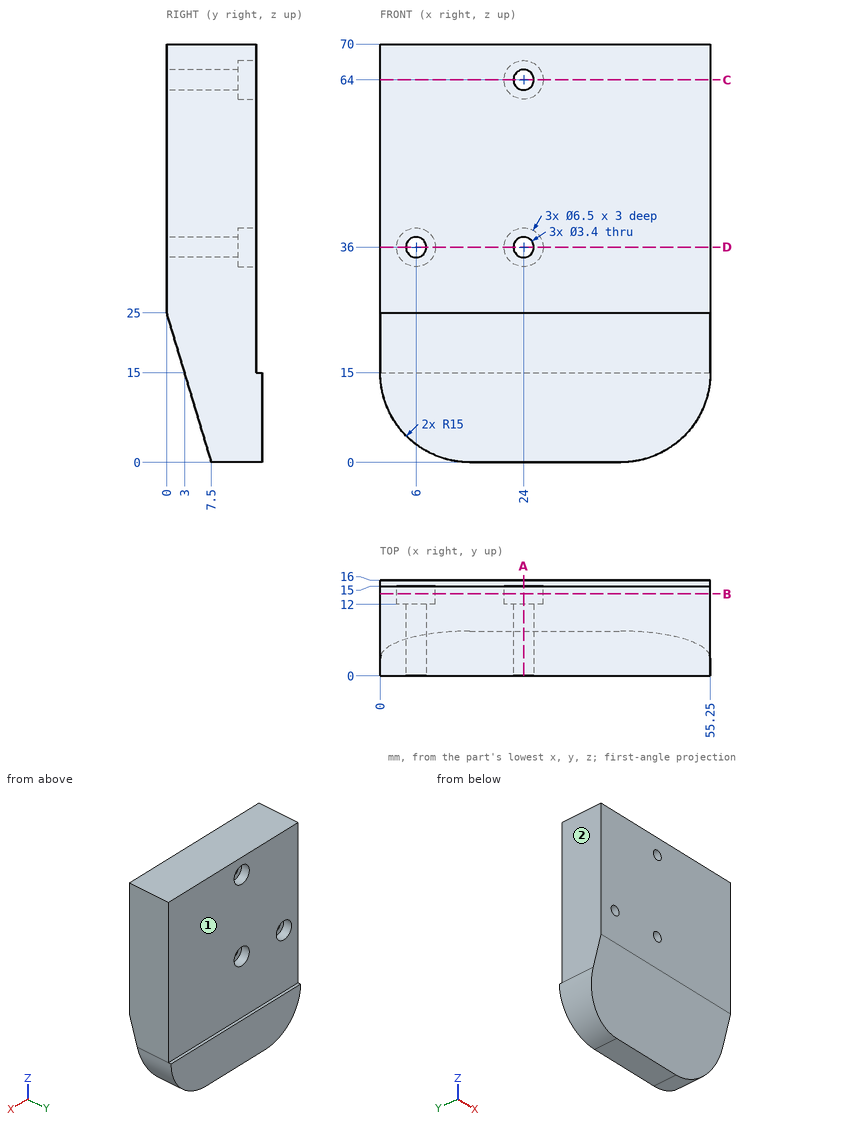
Geometry: see drawing. Coordinates: mm, zero at the bounding-box minimum. A direction names the side the tool comes from. Coordinates: 2 decimals unless noted, no trailing zeros. Write each loop counter-clockwise with the first axis right and the second up, starting at its lowest first coordinate (ties: lowest second). Pieces come first, ordered by that corner, then holes.
1) Pin query (flat end, axial travel): pin 1 Ø2 at (x, z) = (24.5, 35) entering from +Y; pin 2 Ø3 at (x, z) = (24, 64) entering from +Y; pin 3 Ø0.5 at (x, y) = (20, 15.5) entering from +Z; pin 4 Ø3 at (x, z) = (5, 34.5) entering from +Y. Return the tip coordinate at first contact, or that it passes through.
2) Section B-B on y = 13.75. Output: boundary loops of the cut face in (x, z).
3) Section C-C on z = 64. Output: boundary loops of the cut face in (x, y).
4) Material intervals for line 1 along Z through (x, y) = (24, 13.7); line 2 along Z through (x, y) = (24, 8); line 3 along X through (y, z) = (4, 36), sorted ascending.
5) Section A-A on x = 24. Output: boundary loops of the cut face in (y, z), and give its area (3 significant figures).
6) Set-up query: the marked faces 1 and 2. Return all of +Z, -Z, +X, -X, +Y, -Y with unobstructed straight access to the full face (end or side cutting, diameter ignored); none if empty.
7) Section D-D on z = 36. Output: boundary loops of the cut face in (x, y), and give its area (3 significant figures).
Check result:
1. pin 1: stops at y = 12
1. pin 2: passes through
1. pin 3: stops at z = 15
1. pin 4: stops at y = 15
2. outline: (0, 15) arc R15 ccw to (15, 0) - (40.25, 0) arc R15 ccw to (55.25, 15) - (55.25, 70) - (0, 70) - close; hole circle Ø6.5 at (6, 36); hole circle Ø6.5 at (24, 36); hole circle Ø6.5 at (24, 64)
3. outline: (0, 0) - (22.3, 0) - (22.3, 12) - (20.75, 12) - (20.75, 15) - (0, 15) - close; (25.7, 0) - (55.25, 0) - (55.25, 15) - (27.25, 15) - (27.25, 12) - (25.7, 12) - close
4. line 1: z = 0 to 32.75, 39.25 to 60.75, 67.25 to 70
4. line 2: z = 0 to 34.3, 37.7 to 62.3, 65.7 to 70
4. line 3: x = 0 to 4.3, 7.7 to 22.3, 25.7 to 55.25
5. outline: (0, 25) - (7.5, 0) - (16, 0) - (16, 15) - (15, 15) - (15, 32.75) - (12, 32.75) - (12, 34.3) - (0, 34.3) - close; (0, 37.7) - (12, 37.7) - (12, 39.25) - (15, 39.25) - (15, 60.75) - (12, 60.75) - (12, 62.3) - (0, 62.3) - close; (0, 65.7) - (12, 65.7) - (12, 67.25) - (15, 67.25) - (15, 70) - (0, 70) - close
5. area: 851 mm2
6. face 1: +Z, +X, -X, +Y
6. face 2: +Z, -Z, -X, +Y, -Y
7. outline: (0, 0) - (4.3, 0) - (4.3, 12) - (2.75, 12) - (2.75, 15) - (0, 15) - close; (7.7, 0) - (22.3, 0) - (22.3, 12) - (20.75, 12) - (20.75, 15) - (9.25, 15) - (9.25, 12) - (7.7, 12) - close; (25.7, 0) - (55.25, 0) - (55.25, 15) - (27.25, 15) - (27.25, 12) - (25.7, 12) - close
7. area: 708 mm2
